Could you check a few things on this model? Use its own coordinates, in mm. A direction names the side the tool comes from. Coordinates: 2 decimals unless noted, no trailing zeros. Loops run counter-clockwise (first coordinate to the right, second up) from the corner with the lowest first, then second, coordinate; pieces in that order, holes last.
1) Imagine slicing it at A-A on x = 0.75. Please give me the cut outline in (y, z), plus the area to 3 significant figures.
2) Will these pins go through, and if not, where does the flat tip stop? P1, Ø5, axis at x = -1, z = 23, coming from the +Y side; P2, Ø2.5, axis at x = 0.5, z = 26.5, coming from the -Y side.
3) If I drill on line 1 along Z through (x, y) = (1.5, 4.5); line 2 along Y through (x, z) = (0.25, 18.5); line 3 along Y through (x, z) = (3, 24), over which ranges is the centre line in solid material (lowest first)?
4) For faces 1 (the face through (3.48, 1.97, 21.86)), 2 (the face through (0, -4, 22)), 3 (the face through (-3.48, -1.97, 21.86)), which set-ups out of +Z, -Z, +X, -X, +Y, -Y let a thin tool reach every point of the face, with its end or its side?
5) Imagine slicing it at B-B on y = -3.25. Please give me the cut outline in (x, z).
6) Imagine slicing it at C-C on z = 13. Please give me the cut outline in (x, y).
```python
from build123d import *

# Parameters (mm, degrees)
SKETCH_W     = 12.5
SKETCH_H     = 12.5
PAD_DEPTH    = 12
PAD001_DEPTH = 20


with BuildPart() as part:
    # Sketch → Pad (new body)
    with BuildSketch(Plane.XY):
        Rectangle(SKETCH_W, SKETCH_H)
    extrude(amount=PAD_DEPTH)

    # Sketch001 (on Face6 of Pad) → Pad001 (join)
    with BuildSketch(Plane.XY.offset(12)):
        Polygon((-2.309401, 4), (-4.618802, 0), (-2.309401, -4), (2.309401, -4), (4.618802, 0), (2.309401, 4), align=None)
    extrude(amount=PAD001_DEPTH)


solid = part.part
```
Filled in:
1. outline: (-6.25, 0) - (6.25, 0) - (6.25, 12) - (4, 12) - (4, 32) - (-4, 32) - (-4, 12) - (-6.25, 12) - close
1. area: 310 mm2
2. P1: stops at y = 4
2. P2: stops at y = -4
3. line 1: z = 0 to 12
3. line 2: y = -4 to 4
3. line 3: y = -2.8 to 2.8
4. face 1: +Z, +X, +Y
4. face 2: +Z, +X, -X, -Y
4. face 3: +Z, -X, -Y
5. outline: (-6.25, 0) - (6.25, 0) - (6.25, 12) - (2.74, 12) - (2.74, 32) - (-2.74, 32) - (-2.74, 12) - (-6.25, 12) - close
6. outline: (-4.62, 0) - (-2.31, -4) - (2.31, -4) - (4.62, 0) - (2.31, 4) - (-2.31, 4) - close
